```python
from build123d import *

# Parameters (mm, degrees)
F0_R     = 108.15
F0_R_2   = 99.95
F1_DEPTH = 250
F3_R     = 14
F4_REACH = 191.9641662574
F6_R     = 11
F7_REACH = 148.2780486573


with BuildPart() as f1:
    # F0 (on Top) → F1 (new body)
    with BuildSketch(Plane.XY):
        Circle(F0_R)
        Circle(F0_R_2, mode=Mode.SUBTRACT)
    extrude(amount=F1_DEPTH)

    f4_end = f1.faces().sort_by_distance((-108.15, 0, 125))[0]
    # F3 (on face) → F4 (cut, up to a face of the model that its end follows)
    with BuildSketch(Plane(origin=(0, 0, 0), x_dir=(-0.6427876097, -0.7660444431, 0), z_dir=(-0.7660444431, 0.6427876097, 0))):
        with Locations((0, 30)):
            Circle(F3_R)
    f4_long = extrude(amount=-F4_REACH, mode=Mode.PRIVATE)
    add(split(f4_long, bisect_by=f4_end, keep=Keep.BOTTOM, mode=Mode.PRIVATE), mode=Mode.SUBTRACT)

    f7_end = f1.faces().sort_by_distance((-108.15, 0, 125))[0]
    # F6 (on face) → F7 (cut, up to a face of the model that its end follows)
    with BuildSketch(Plane(origin=(0, 0, 0), x_dir=(-0.0871557427, -0.9961946981, 0), z_dir=(-0.9961946981, 0.0871557427, 0))):
        with Locations((0, 120)):
            Circle(F6_R)
    f7_long = extrude(amount=-F7_REACH, mode=Mode.PRIVATE)
    add(split(f7_long, bisect_by=f7_end, keep=Keep.BOTTOM, mode=Mode.PRIVATE), mode=Mode.SUBTRACT)


solid = f1.part
```
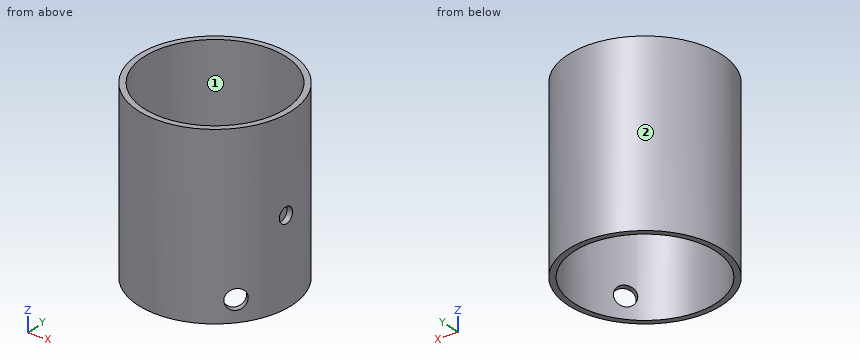
CAD build for the part. Positions are in the model's coordinates, mm. Face numbers are marked on the shaded views. Give positions to 0.01 mm unless a question says otherwise; leave off trailing zeros. Loops run counter-clockwise (first coordinate to the right, second up) from the corner with the lowest first, then second, coordinate; pieces in that order, holes last. Notation, with made-up numbers: (-7, 15.5) -> (11, 15.5) arc R32 ccw to (11, 53.5) -> close; hole circle Ø8 at (-12.5, -26.75). An arc over 180 degrees is marked (long way). Use a Markdown table: item, result.
1. Mould opens along Y. For the marked faces 1 and 2 say: pulls with the +Y half, pulls with the -Y half, needs draft (parallel to the pull), parting line crosses it, or undercut.
Check result:
| item | result |
|---|---|
| face 1 | undercut |
| face 2 | parting line crosses it |
2. Flat gauge pins, fed straight in: pin 1 (8 mm diameter, centred on x = 25.5, z = 162, fed in from +Y); pin 2 (2 mm diameter, centred on x = -31.5, z = 181.5, fed in from +Y); pin 3 (5 mm diameter, centred on x = 81, z = 171.5, fed in from +Y). Where does each tip first touch, or does it go through?
Check result:
| item | result |
|---|---|
| pin 1 | stops at y = 105.99 |
| pin 2 | stops at y = 103.76 |
| pin 3 | stops at y = 74.39 |
3. Slice it at B-B (y = 69). List the corners of the cut face in (x, z), plus the area to 3 significant figures.
Check result:
| item | result |
|---|---|
| outline | (-83.28, 0) -> (-72.31, 0) -> (-72.31, 250) -> (-83.28, 250) -> close; (72.31, 0) -> (83.28, 0) -> (83.28, 250) -> (72.31, 250) -> close |
| area | 5,480 mm^2 |
4. Wall check: L1, parallel to X at y = -3, z = 142; L2, parallel to Y at x = -1, z = 36 (3 decimals); L3, parallel to Y at x = -30, z = 116. Give the ranges that are in metal, low to high. Write a range as [from, to].
Check result:
| item | result |
|---|---|
| L1 | x = [-108.11, -99.9], [99.9, 108.11] |
| L2 | y = [-108.145, -99.945], [99.945, 108.145] |
| L3 | y = [-103.91, -95.34], [95.34, 103.91] |
5. Slice it at A-A (x = 0). List the corners of the cut face in (y, z).
Check result:
| item | result |
|---|---|
| outline | (-108.15, 0) -> (-99.95, 0) -> (-99.95, 250) -> (-108.15, 250) -> close; (99.95, 0) -> (108.15, 0) -> (108.15, 250) -> (99.95, 250) -> close |
6. Slice it at C-C (z = 144). List the corners of the cut face in (x, y).
Check result:
| item | result |
|---|---|
| outline | circle Ø216.3 at (0, 0); hole circle Ø199.9 at (0, 0) |
7. Slice it at D-D (y = -6.5). Give the number of separate pieces and of enclosed holes in the cut face, plus the area to 3 significant figures.
Check result:
| item | result |
|---|---|
| separate pieces | 3 |
| enclosed holes | 0 |
| area | 3,930 mm^2 |
